from build123d import *

# Parameters (mm, degrees)
SKETCH2_W               = 33
SKETCH2_H               = 28
BOSS_EXTRUDE1_DEPTH     = 46
CUT_EXTRUDE1_DEPTH      = 59.318093247
CUT_EXTRUDE1_DEPTH_BACK = 59.318093247
SKETCH3_W               = 41
SKETCH3_H               = 17.5
BOSS_EXTRUDE2_DEPTH     = 3
BOSS_EXTRUDE3_DEPTH     = 27
FILLET2_START           = -3.5
FILLET2_DEPTH           = 4.654998639
FILLET2_START_2         = -13.5
FILLET2_2_DEPTH         = 27
FILLET3_R               = 16.5
FILLET4_R               = 6
SKETCH6_W               = 13
SKETCH6_H               = 23
CUT_EXTRUDE2_DEPTH      = 9
SKETCH7_R               = 6.5
CUT_EXTRUDE3_DEPTH      = 9
SKETCH8_R               = 1.15
CUT_EXTRUDE4_DEPTH      = 8
SKETCH9_R               = 1.3
SKETCH9_R_2             = 2.5
CUT_EXTRUDE5_DEPTH      = 47.360004954


with BuildPart() as part:
    # Sketch2 → Boss-Extrude1 (new body)
    with BuildSketch(Plane.XY):
        Rectangle(SKETCH2_W, SKETCH2_H)
    extrude(amount=BOSS_EXTRUDE1_DEPTH)

    # Sketch3 → Cut-Extrude1 (cut, two sides: drawn at the far end of the back side and taken through both)
    with BuildSketch(Plane.ZY.offset(16.5).offset(-CUT_EXTRUDE1_DEPTH_BACK)):
        with Locations((25.5, 5.25)):
            Rectangle(SKETCH3_W, SKETCH3_H)
    extrude(amount=CUT_EXTRUDE1_DEPTH + CUT_EXTRUDE1_DEPTH_BACK, mode=Mode.SUBTRACT)

    # Sketch4 → Boss-Extrude2 (add)
    with BuildSketch(Plane.ZY.offset(16.5)):
        with BuildLine():
            Line((46, -2), (46, -3.5))
            Line((46, -3.5), (5, -3.5))
            Line((5, -3.5), (5, 14))
            add(Edge.make_bspline(
                [(5, 14), (15.432246661, 2.101110375), (46, -2)],
                knots=[0, 0, 0, 1, 1, 1], degree=2))
        make_face()
    boss_extrude2 = extrude(amount=-BOSS_EXTRUDE2_DEPTH)

    # Mirror1: Boss-Extrude2 across plane
    add(boss_extrude2.mirror(Plane(origin=(0, 0, 0), x_dir=(0, 0, 1), z_dir=(1, 0, 0))))

    # Sketch5 → Boss-Extrude3 (add)
    with BuildSketch(Plane(origin=(-13.5, 0, 0), x_dir=(0, 0, -1), z_dir=(1, 0, 0))):
        with BuildLine():
            Line((-46, -3.5), (-43, -3.5))
            Line((-43, -3.5), (-43, -1.57137225))
            add(Edge.make_bspline(
                [(-43, -1.57137225), (-44.474940132, -1.795390955), (-46.000000067, -2.000000009)],
                knots=[0.950108864, 0.950108864, 0.950108864, 1, 1, 1], degree=2))
            Line((-46.000000067, -2.000000009), (-46, -3.5))
        make_face()
    extrude(amount=BOSS_EXTRUDE3_DEPTH)

    # Fillet2: read off the stored shape, not the designer's step
    # Fillet2 outline → Fillet2 (add)
    with BuildSketch(Plane(origin=(0, 0, 0), x_dir=(1, 0, 0), z_dir=(0, 1.0, -9.82210297214819e-12)).offset(FILLET2_START)):
        with BuildLine():
            Line((13.5, -43.00000001), (13.5, -29.5))
            ThreePointArc((13.5, -29.5), (9.545941546, -39.045941546), (0, -43))
            Line((0, -43), (13.5, -43.00000001))
        make_face()
        with BuildLine():
            Line((-13.5, -43), (0, -43))
            ThreePointArc((0, -43), (-9.545941546, -39.045941546), (-13.5, -29.5))
            Line((-13.5, -29.5), (-13.5, -43))
        make_face()
    extrude(amount=FILLET2_DEPTH)

    # Fillet2 2 outline → Fillet2 2 (cut)
    with BuildSketch(Plane.YZ.offset(FILLET2_START_2)):
        with BuildLine():
            Line((1.154998639, 43.000000001), (-1.57137225, 43.000000001))
            add(Edge.make_bspline(
                [(-1.57137225, 43.000000001), (-0.450949941, 35.623134616), (1.154998546, 29.499999976)],
                knots=[0.049891135, 0.049891135, 0.049891135, 0.299420037, 0.299420037, 0.299420037], degree=2))
            Line((1.154998546, 29.499999976), (1.154998639, 43.000000001))
        make_face()
    extrude(amount=FILLET2_2_DEPTH, mode=Mode.SUBTRACT)

    # Fillet3
    # the kernel refuses this fillet: 16.5 mm, written as the material it takes off along each edge
    with BuildSketch(Plane(origin=(-16.5, -55.25, 46), x_dir=(0, 0, -1), z_dir=(0, 1, 0)), Plane(origin=(16.5, 39.25, 46), x_dir=(0, 0, -1), z_dir=(0, -1, 0))) as fillet3_piece_1:
        with BuildLine():
            CenterArc((FILLET3_R, -FILLET3_R), FILLET3_R, 90, 90)
            Line((0, -FILLET3_R), (0, 0))
            Line((0, 0), (FILLET3_R, 0))
        make_face()
    extrude(amount=94.5, mode=Mode.SUBTRACT)

    # Fillet4
    # the kernel refuses this fillet: 6 mm, written as the material it takes off along each edge
    with BuildSketch(Plane(origin=(-16.5, 14, -15), x_dir=(1, 0, 0), z_dir=(0, 0, 1))) as fillet4_piece_1:
        with BuildLine():
            CenterArc((FILLET4_R, -FILLET4_R), FILLET4_R, 90, 90)
            Line((0, -FILLET4_R), (0, 0))
            Line((0, 0), (FILLET4_R, 0))
        make_face()
    extrude(amount=35, mode=Mode.SUBTRACT)
    with BuildSketch(Plane(origin=(16.5, 14, -15), x_dir=(-1, 0, 0), z_dir=(0, 0, 1))) as fillet4_piece_2:
        with BuildLine():
            CenterArc((FILLET4_R, FILLET4_R), FILLET4_R, 180, 90)
            Line((0, FILLET4_R), (0, 0))
            Line((0, 0), (FILLET4_R, 0))
        make_face()
    extrude(amount=35, mode=Mode.SUBTRACT)

    # Sketch6 → Cut-Extrude2 (cut)
    with BuildSketch(Plane(origin=(0, -3.5, 0), x_dir=(1, 0, 0), z_dir=(0, 1, 0))):
        with Locations((0, -23)):
            Rectangle(SKETCH6_W, SKETCH6_H)
    extrude(amount=-CUT_EXTRUDE2_DEPTH, mode=Mode.SUBTRACT)

    # Sketch7 → Cut-Extrude3 (cut)
    with BuildSketch(Plane(origin=(0, -12.5, 0), x_dir=(1, 0, 0), z_dir=(0, 1, 0))):
        with Locations(Location((0, -28, 0), (0, 0, 270))):
            Circle(SKETCH7_R)
    extrude(amount=-CUT_EXTRUDE3_DEPTH, mode=Mode.SUBTRACT)

    # Sketch8 → Cut-Extrude4 (cut)
    with BuildSketch(Plane(origin=(0, -3.5, 0), x_dir=(1, 0, 0), z_dir=(0, 1, 0))):
        with Locations(Location((0, -9.2, 0), (0, 0, 180))):
            Circle(SKETCH8_R)
        with Locations(Location((0, -36.8, 0), (0, 0, 180))):
            Circle(SKETCH8_R)
    extrude(amount=-CUT_EXTRUDE4_DEPTH, mode=Mode.SUBTRACT)

    # Sketch9 → Cut-Extrude5 (cut, through all)
    with BuildSketch(Plane.XY.offset(5)):
        with Locations((0.5, 0)):
            Circle(SKETCH9_R)
        with Locations((5, 0)):
            Circle(SKETCH9_R_2)
        with Locations((9.5, 0)):
            Circle(SKETCH9_R)
    extrude(amount=-CUT_EXTRUDE5_DEPTH, mode=Mode.SUBTRACT)


solid = part.part
Read the model definition and answer for the solid it produces. Units are mm, in the model's axes. A direction names the side the tool comes from. Round coordinates to 2 decimals unless told otherwise and drop trailing zeros. Order: outer loops, then holes, each group sorted by start corner. A loop starts at its lowest first (then second) coordinate and runs counter-clockwise, first axis right, second up.
1) The part is cut by section A-A on y = -10. Write down the section's boundary in (x, z), plus the area to 3 significant figures.
2) For faces 1 (the face through (10.74, 0.39, 2.54)), 2 (the face through (-16.5, -3, 15)), 3 (the face through (0, -8, 11.5)), determine the directions among +Z, -Z, +X, -X, +Y, -Y from which every point of the face is accessible in a straight line to the end or side of a thin tool.
3) Straight lines are drawn through the part: L1, parallel to Z at x = 0, y = -5.5; L2, parallel to Y at x = 0.5, z = 1.45; L3, parallel to X at y = -11.75, z = 22.5. For each, find the intervals that lie inside material, in ascending order.
4) The part is cut by section B-B on y = 0. Give the number of separate pieces and of enclosed holes in the cut face, plus the area to 3 significant figures.
5) The mould has two halves that part along X. Classify faces 4 (the face through (16.5, -3, 15)), 5 (the face through (-0.53, -7.44, 8.18)), 6 (the face through (0, -3, 0)), 7 (the face through (-15.377, 11.495, 3.34)): released by +X, released by -X, zero draft, split by the parting line, or undercut.
6) Flat-ended cylindrical pins translate along their axes: pin 1 (1.6 mm diameter, centred on x = 0.5, y = 0, fed in from +Z); pin 2 (13.5 mm diameter, centred on x = 4, z = 22.5, fed in from +Y); pin 3 (1.5 mm diameter, centred on x = -11, y = 1.5, fed in from +Z); pin 4 (1.5 mm diameter, centred on x = -1.5, y = -5, fed in from +Z). Find the tip coordinate at first contact, or state that the pin passes through.
Resolved:
1. outline: (-16.5, 0) - (16.5, 0) - (16.5, 29.5) arc R16.5 ccw to (-16.5, 29.5) - close; hole (-6.5, 11.5) - (6.5, 11.5) - (6.5, 34.5) - (-6.5, 34.5) - close; hole circle Ø2.3 at (0, 9.2); hole circle Ø2.3 at (0, 36.8)
1. area: 1,090 mm2
2. face 1: -Z
2. face 2: +Z, -Z, -X, +Y, -Y
2. face 3: +Y
3. L1: z = 0 to 8.05, 10.35 to 11.5, 34.5 to 35.65, 37.95 to 46
3. L2: y = -14 to -1.3, 1.3 to 14
3. L3: x = -16.5 to -6.5, 6.5 to 16.5
4. separate pieces: 4
4. enclosed holes: 0
4. area: 291 mm2
5. face 4: released by +X
5. face 5: undercut
5. face 6: zero draft
5. face 7: released by -X
6. pin 1: passes through
6. pin 2: stops at y = -3.5
6. pin 3: stops at z = 5
6. pin 4: stops at z = 45.98
